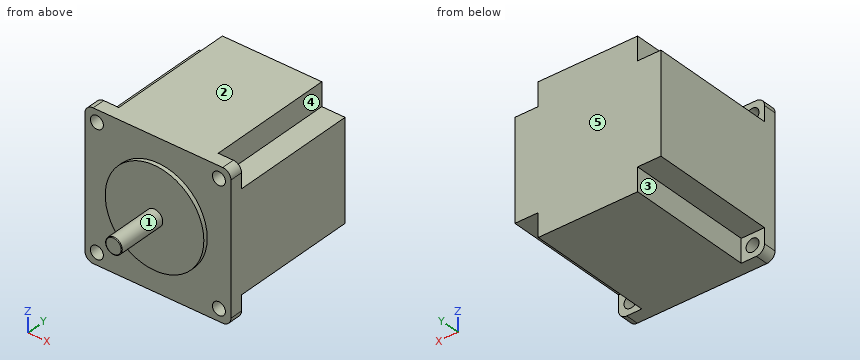
Autodesk Inventor part; units mm, degrees
ref_plane "YZ Plane" through (0, 0, 0) normal (1, 0, 0) x (0, 1, 0)
ref_plane "XZ Plane" through (0, 0, 0) normal (0, 1, 0) x (-1, 0, 0)
ref_plane "XY Plane" through (0, 0, 0) normal (0, 0, 1) x (1, 0, 0)
sketch "Sketch1" plane through (0, 0, 0) normal (0, 1, 0) x (-1, 0, 0)
  line L0 (-28.2, -28.2) -> (28.2, -28.2)
  line L1 (28.2, -28.2) -> (28.2, 28.2)
  line L2 (28.2, 28.2) -> (-28.2, 28.2)
  line L3 (-28.2, 28.2) -> (-28.2, -28.2)
  line L4 (-28.2, -28.2) -> (28.2, 28.2) construction
  line L5 (28.2, -28.2) -> (-28.2, 28.2) construction
  line L6 (28.2, 28.2) -> (19.2, 28.2)
  line L7 (19.2, 28.2) -> (19.2, 19.2)
  line L8 (19.2, 19.2) -> (28.2, 19.2)
  line L9 (28.2, 19.2) -> (28.2, 28.2)
  line L10 (15.7012, 0) -> (-14.7312, 0)
  line L11 (0, 21.5613) -> (0, -24.5212)
  line L12 (28.2, -28.2) -> (19.2, -28.2)
  line L13 (19.2, -28.2) -> (19.2, -19.2)
  line L14 (19.2, -19.2) -> (28.2, -19.2)
  line L15 (28.2, -19.2) -> (28.2, -28.2)
  line L16 (-28.2, 28.2) -> (-19.2, 28.2)
  line L17 (-19.2, 28.2) -> (-19.2, 19.2)
  line L18 (-19.2, 19.2) -> (-28.2, 19.2)
  line L19 (-28.2, 19.2) -> (-28.2, 28.2)
  line L20 (-28.2, -28.2) -> (-19.2, -28.2)
  line L21 (-19.2, -28.2) -> (-19.2, -19.2)
  line L22 (-19.2, -19.2) -> (-28.2, -19.2)
  line L23 (-28.2, -19.2) -> (-28.2, -28.2)
  circle A0 centre (23.57, 23.57) radius 2.5
  circle A1 centre (23.57, -23.57) radius 2.5
  circle A2 centre (-23.57, 23.57) radius 2.5
  circle A3 centre (-23.57, -23.57) radius 2.5
  point P0 (0, 0)
  point P1 (0, 0)
  point P2 (0, 0)
  dimension "d0" = 56.4
  dimension "d1" = 56.4
  dimension "d2" = 9
  dimension "d3" = 9
  dimension "d6" = 47.14
  dimension "d7" = 47.14
  dimension "d8" = 5
extrude "Extrusion1" add sketch "Sketch1" along normal blind 54 contours L21 L22 L3 L18 L17 L2 L7 L8 L1 L14 L13 L0
extrude "Extrusion2" add sketch "Sketch1" along normal blind 5 contours L3 L22 L21 L0 | L13 L14 L1 L0 | L3 L2 L17 L18 | L8 L7 L2 L1
fillet "Fillet1" radius 3.175 4 edges at (-28.2, 2.5, 28.2) (-28.2, 2.5, -28.2) (28.2, 2.5, -28.2) (28.2, 2.5, 28.2)
sketch "Sketch2" plane through (0, 0, 0) normal (0, -1, 0) x (1, 0, 0)
  circle A0 centre (0, 0) radius 19.05
  dimension "d12" = 38.1
extrude "Extrusion3" add sketch "Sketch2" along normal blind 1.6
sketch "Sketch3" plane through (0, 0, 0) normal (0, -1, 0) x (1, 0, 0)
  circle A0 centre (0, 0) radius 3.175
  dimension "d15" = 6.35
extrude "Extrusion4" add sketch "Sketch3" along normal blind 21
fillet "Fillet2" radius 0.254 1 edges at (-3.175, -21, 0)
equation "\"d1\" = d0"
equation "\"d3\" = d2"
equation "\"d7\" = d6"
properties part number "Stepper_Motor_Large"
Part model, mm, in its own coordinate system. Face numbers are marked on the shaded views. A direction names the side the tool comes from. Coordinates: 2 decimals unless noted, no trailing zeros. Order: outer loops, then holes, each group sorted by start corner. A loop starts at its lowest first (then second) coordinate and runs counter-clockwise, first axis right, second up. Notation, with made-up numbers: (60.25, 33.25) -> (76.25, 33.25) arc R4 ccw to (76.25, 39.25) -> close; hole circle Ø4 at (18, 53.5). An arc over 180 degrees is marked (long way). Put each result on its own line as item: value. Start each with the question number.
(1) Band-saw the part on D-D (x = 0). Give the cut face in (y, z) (3 decimals), then the cut area to 3 significant figures.
(2) Pin check, flat tips, straight feed: pin 1 Ø3 at (x, z) = (7, 15.5) entering from -Y; pin 2 Ø8 at (x, z) = (-23.57, -23.57) entering from +Y; pin 3 Ø10 at (x, y) = (-24.5, 24) entering from -Z. Stop position of each tip, or through.
(3) Band-saw the part on C-C (y = 17.5). Give the cut face in (x, z).
(4) Which spindle directions (+Z, -Z, +X, -X, +Y, -Y) get a long thin tool onto all of the face, cutting with end or side? Do the marked faces 1, 2, 3, 4 and 5. Say none if no direction does.
(5) Probe line 1 along Z through (x, y) = (23.57, 3.05); line 2 along X through (y, z) = (1, 23); line 3 along Y through (x, z) = (-2.5, -4.5). List the from-to ranges inside material, lowest first. Write a range as [from, to].
(6) Band-saw the part on A-A (z = 23.57). Give the cut face in (x, y), then the cut area to 3 significant figures.
(7) Band-saw the part on B-B (x = 23.57). Give the cut face in (y, z), then the cut area to 3 significant figures.
Determined:
1. outline: (-21, -2.921) arc R0.254 ccw to (-20.746, -3.175) -> (-1.6, -3.175) -> (-1.6, -19.05) -> (0, -19.05) -> (0, -28.2) -> (54, -28.2) -> (54, 28.2) -> (0, 28.2) -> (0, 19.05) -> (-1.6, 19.05) -> (-1.6, 3.175) -> (-20.746, 3.175) arc R0.254 ccw to (-21, 2.921) -> close
1. area: 3,230 mm²
2. pin 1: stops at y = -1.6
2. pin 2: stops at y = 5
2. pin 3: stops at z = -19.2
3. outline: (-28.2, -19.2) -> (-19.2, -19.2) -> (-19.2, -28.2) -> (19.2, -28.2) -> (19.2, -19.2) -> (28.2, -19.2) -> (28.2, 19.2) -> (19.2, 19.2) -> (19.2, 28.2) -> (-19.2, 28.2) -> (-19.2, 19.2) -> (-28.2, 19.2) -> close
4. face 1: -Y
4. face 2: +Z, +X, -X, +Y, -Y
4. face 3: -Z, -X, +Y
4. face 4: +Z, +X, +Y
4. face 5: +Z, -Z, +X, -X, +Y
5. line 1: z = [-28.2, -26.07], [-21.07, 21.07], [26.07, 28.2]
5. line 2: x = [-28.2, -26], [-21.14, 21.14], [26, 28.2]
5. line 3: y = [-1.6, 54]
6. outline: (-28.2, 0) -> (-26.07, 0) -> (-26.07, 5) -> (-28.2, 5) -> close; (-21.07, 0) -> (21.07, 0) -> (21.07, 5) -> (19.2, 5) -> (19.2, 54) -> (-19.2, 54) -> (-19.2, 5) -> (-21.07, 5) -> close; (26.07, 0) -> (28.2, 0) -> (28.2, 5) -> (26.07, 5) -> close
6. area: 2,110 mm²
7. outline: (0, -28.2) -> (5, -28.2) -> (5, -26.07) -> (0, -26.07) -> close; (0, -21.07) -> (5, -21.07) -> (5, -19.2) -> (54, -19.2) -> (54, 19.2) -> (5, 19.2) -> (5, 21.07) -> (0, 21.07) -> close; (0, 26.07) -> (5, 26.07) -> (5, 28.2) -> (0, 28.2) -> close
7. area: 2,110 mm²
